```python
from build123d import *

# Parameters (mm, degrees)
SKETCH1_W           = 100
SKETCH1_H           = 200
BOSS_EXTRUDE1_DEPTH = 35
SKETCH2_R           = 4
CUT_EXTRUDE1_DEPTH  = 30
SKETCH3_R           = 5
CUT_EXTRUDE2_DEPTH  = 210.105236663
SKETCH4_W           = 20
SKETCH4_H           = 50
CUT_EXTRUDE3_DEPTH  = 118.153745139
SKETCH6_R           = 8.1
CUT_EXTRUDE4_DEPTH  = 5
SKETCH7_W           = 30
SKETCH7_H           = 50
CUT_EXTRUDE5_DEPTH  = 5


with BuildPart() as part:
    # Sketch1 → Boss-Extrude1 (new body)
    with BuildSketch(Plane.XY):
        Rectangle(SKETCH1_W, SKETCH1_H)
    extrude(amount=BOSS_EXTRUDE1_DEPTH)

    # Sketch2 → Cut-Extrude1 (cut)
    with BuildSketch(Plane.XY.offset(35)):
        with Locations((-30, 10)):
            Circle(SKETCH2_R)
        with Locations((30, 10)):
            Circle(SKETCH2_R)
    extrude(amount=-CUT_EXTRUDE1_DEPTH, mode=Mode.SUBTRACT)

    # Sketch3 → Cut-Extrude2 (cut, through all)
    with BuildSketch(Plane(origin=(0, 100, 0), x_dir=(1, 0, 0), z_dir=(0, 1, 0))):
        with Locations(Location((0, -10, 0), (0, 0, 270))):
            Circle(SKETCH3_R)
    extrude(amount=-CUT_EXTRUDE2_DEPTH, mode=Mode.SUBTRACT)

    # Sketch4 → Cut-Extrude3 (cut, through all)
    with BuildSketch(Plane(origin=(0, 0, 0), x_dir=(-1, 0, 0), z_dir=(0, 0, -1))):
        with Locations((0, 40)):
            Rectangle(SKETCH4_W, SKETCH4_H)
    extrude(amount=-CUT_EXTRUDE3_DEPTH, mode=Mode.SUBTRACT)

    # Sketch6 → Cut-Extrude4 (cut)
    with BuildSketch(Plane(origin=(0, 100, 0), x_dir=(1, 0, 0), z_dir=(0, 1, 0))):
        with Locations(Location((0, -10, 0), (0, 0, 270))):
            Circle(SKETCH6_R)
    cut_extrude4 = extrude(amount=-CUT_EXTRUDE4_DEPTH, mode=Mode.SUBTRACT)

    # Mirror1: Cut-Extrude4 across plane
    add(cut_extrude4.mirror(Plane.ZX), mode=Mode.SUBTRACT)

    # Sketch7 → Cut-Extrude5 (cut)
    with BuildSketch(Plane.XY.offset(35)):
        with Locations((0, 40)):
            Rectangle(SKETCH7_W, SKETCH7_H)
    extrude(amount=-CUT_EXTRUDE5_DEPTH, mode=Mode.SUBTRACT)


solid = part.part
```
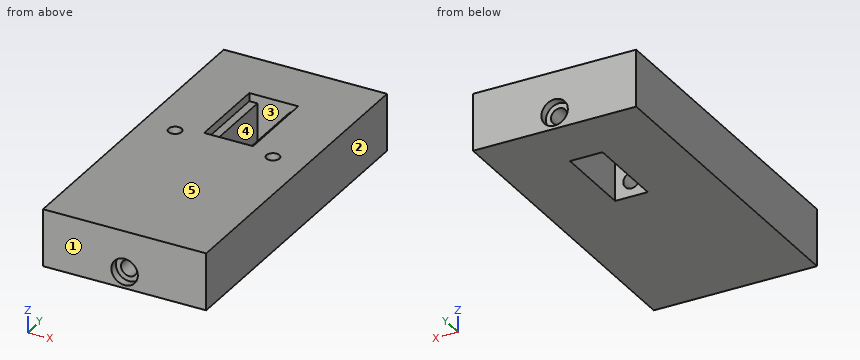
Verification items for the finished model (mm, model axes). Face numbers are marked on the shaded views. A direction names the side the tool comes from. Coordinates: 2 decimals unless noted, no trailing zeros. Loops run counter-clockwise (first coordinate to the right, second up) from the corner with the lowest first, then second, coordinate; pieces in that order, holes last. Notation, with made-up numbers: (27.5, -38.5) - (51.5, -38.5) arc R24 cw to (51.5, -1.5) - close; hole circle Ø7 at (35, 88.25). An arc over 180 degrees is marked (long way). Answer as a JSON object with one key per item and string values.
(1) Cross-section at D-D, the plane z = 26. Record the boundary of the cut face in (x, y), then the cut area to 3 significant figures.
Response:
{"outline": "(-50, -100) - (50, -100) - (50, 100) - (-50, 100) - close; hole circle Ø8 at (-30, 10); hole (-10, 15) - (10, 15) - (10, 65) - (-10, 65) - close; hole circle Ø8 at (30, 10)", "area": "18,900 mm²"}
(2) Mould release check, pull along Y, two halves, no side actions. Record for the marked faces 1, 2 and 3: pulls with the +Y half, pulls with the -Y half, needs draft (parallel to the pull), parting line crosses it, or undercut.
Response:
{"face 1": "pulls with the -Y half", "face 2": "needs draft", "face 3": "undercut"}
(3) Access from +Z, -Z, +X, -X, +Y, -Y to the whole of each face (thin tool, end or side, straight path). Record for the marked faces 4 and 5.
Response:
{"face 4": "+Z, -Z", "face 5": "+Z, +X, -X, +Y, -Y"}
(4) Cross-section at C-C, the plane y = 10. Record the boundary of the cut face in (x, z).
Response:
{"outline": "(-50, 0) - (50, 0) - (50, 35) - (34, 35) - (34, 5) - (26, 5) - (26, 35) - (-26, 35) - (-26, 5) - (-34, 5) - (-34, 35) - (-50, 35) - close; hole circle Ø10 at (0, 10)"}
(5) Go/stop test with flat-tipped pins: pin 1 Ø3 at (x, z) = (-5.5, 9) entering from -Y; pin 2 Ø6 at (x, z) = (0, 10) entering from +Y; pin 3 Ø8 at (x, z) = (-0.5, 8.5) entering from +Y; pin 4 Ø4 at (x, y) = (-29, 10) entering from +Z. Record where each tip stops, or that it passes through.
Response:
{"pin 1": "stops at y = -95", "pin 2": "passes through", "pin 3": "stops at y = 95", "pin 4": "stops at z = 5"}
(6) Scan lines: line 1 along X through (y, z) = (7, 7.5); line 2 along Y through (x, z) = (-30, 15.25); line 3 along Y through (x, z) = (1, 24). Record each from-to range of solid material in increasing order.
Response:
{"line 1": "x = -50 to -32.65, -27.35 to -4.33, 4.33 to 27.35, 32.65 to 50", "line 2": "y = -100 to 6, 14 to 100", "line 3": "y = -100 to 15, 65 to 100"}
(7) Cross-section at B-B, the plane x = 0. Record the boundary of the cut face in (y, z).
Response:
{"outline": "(-100, 0) - (15, 0) - (15, 5) - (-95, 5) - (-95, 1.9) - (-100, 1.9) - close; (-100, 18.1) - (-95, 18.1) - (-95, 15) - (15, 15) - (15, 35) - (-100, 35) - close; (65, 0) - (100, 0) - (100, 1.9) - (95, 1.9) - (95, 5) - (65, 5) - close; (65, 15) - (95, 15) - (95, 18.1) - (100, 18.1) - (100, 35) - (65, 35) - close"}
(8) Cross-section at A-A, the plane z = 10. Record the boundary of the cut face in (x, y).
Response:
{"outline": "(-50, -100) - (-8.1, -100) - (-8.1, -95) - (-5, -95) - (-5, 15) - (-10, 15) - (-10, 65) - (-5, 65) - (-5, 95) - (-8.1, 95) - (-8.1, 100) - (-50, 100) - close; (5, -95) - (8.1, -95) - (8.1, -100) - (50, -100) - (50, 100) - (8.1, 100) - (8.1, 95) - (5, 95) - (5, 65) - (10, 65) - (10, 15) - (5, 15) - close; hole circle Ø8 at (-30, 10); hole circle Ø8 at (30, 10)"}
